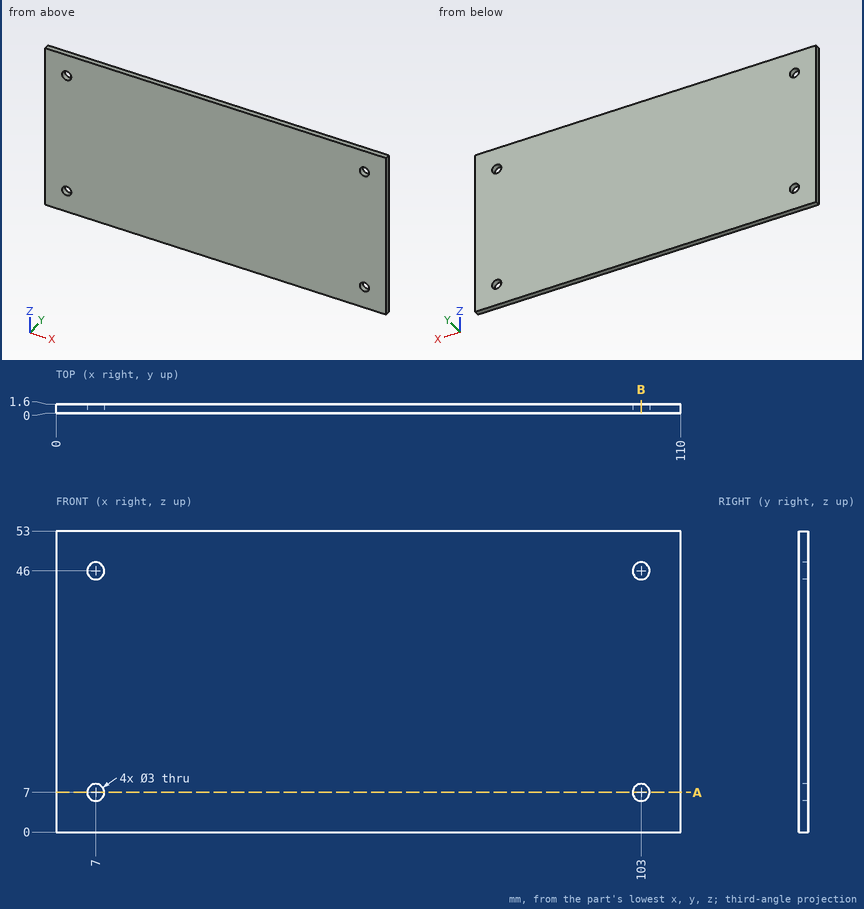
Could you check a few things on this drawing? It's one solid part, dimensions in mm from its lowest x, y, z. Coordinates: 2 decimals unless noted, no trailing zeros. Order: outer loops, then holes, each group sorted by start corner. A loop starts at its lowest first (then second) coordinate and runs counter-clockwise, first axis right, second up.
1. I'm going to push a flat-ended pin straight in: pin 1 (2.5 mm diameter, centred on x = 7, z = 7, fed in from -Y). Where does the tip first touch, or does it pass through?
2. I need wall thicknesses on line 1 (Z direction, x = 103, y = 0.4); line 2 (X direction, y = 1.15, z = 46). Which ranges of each line are inside material? Lowest first, please.
3. If we section it at A-A (z = 7): Please give me the cut outline in (x, y), then the cut area to 3 significant figures.
4. If we section it at B-B (x = 103): Please give me the cut outline in (y, z), then the cut area to 3 significant figures.
Entries:
1. pin 1: passes through
2. line 1: z = 0 to 5.5, 8.5 to 44.5, 47.5 to 53
2. line 2: x = 0 to 5.5, 8.5 to 101.5, 104.5 to 110
3. outline: (0, 0) - (5.5, 0) - (5.5, 1.6) - (0, 1.6) - close; (8.5, 0) - (101.5, 0) - (101.5, 1.6) - (8.5, 1.6) - close; (104.5, 0) - (110, 0) - (110, 1.6) - (104.5, 1.6) - close
3. area: 166 mm2
4. outline: (0, 0) - (1.6, 0) - (1.6, 5.5) - (0, 5.5) - close; (0, 8.5) - (1.6, 8.5) - (1.6, 44.5) - (0, 44.5) - close; (0, 47.5) - (1.6, 47.5) - (1.6, 53) - (0, 53) - close
4. area: 75.2 mm2
